Autodesk Inventor part; units mm, degrees
ref_plane "Work Plane1" through (0, 50.8, 0) normal (0, 1, 0) x (-1, 0, 0)
ref_plane "YZ Plane" through (0, 0, 0) normal (1, 0, 0) x (0, 1, 0)
ref_plane "XY Plane" through (0, 0, 0) normal (0, 0, 1) x (1, 0, 0)
sketch "Sketch1" plane through (0, 0, 0) normal (0, 0, 1) x (1, 0, 0)
  circle A0 centre (0, 0) radius 50.8
  circle A1 centre (0, 0) radius 47.625
  dimension "d0" = 101.6
  dimension "d1" = 95.25
extrude "Extrusion1" add sketch "Sketch1" along normal blind 711.2
ref_plane "Work Plane1" through (0, 50.8, 0) normal (0, 1, 0) x (-1, 0, 0)
sketch "Sketch3" plane through (0, 50.8, 0) normal (0, 1, 0) x (-1, 0, 0)
  line L0 (0, 0) -> (0, 111.76)
  line L1 (-4.7625, 111.76) -> (4.7625, 111.76)
  line L2 (4.7625, 111.76) -> (4.7625, 172.085)
  line L3 (4.7625, 172.085) -> (-4.7625, 172.085)
  line L4 (-4.7625, 172.085) -> (-4.7625, 111.76)
  dimension "d4" = 111.76
  dimension "d5" = 60.325
  dimension "d6" = 9.525
  dimension "d7" = 4.7625
extrude "Extrusion2" cut sketch "Sketch3" against normal blind 25.4
fillet "Fillet1" radius 4.7625 4 edges at (-4.7625, 48.9813, 111.76) (4.7625, 48.9813, 111.76) (4.7625, 48.9813, 172.085) (-4.7625, 48.9813, 172.085)
equation "\"d7\" = 0.5 * d6"
properties part number "PrimaryHullLexanTube_01" material "Polycarbonate, Clear"
Geometry check sheet. Reference: the model listing, model coordinates, mm. Give positions to 0.01 mm unless a question says otherwise; leave off trailing zeros. Loops run counter-clockwise (first coordinate to the right, second up) from the corner with the lowest first, then second, coordinate; pieces in that order, holes last. Notation, with made-up numbers: M 34.5,43.25 L 69.5,43.25 A22 cw 69.5,76.25 Z; hole C 27.25,3.5 d9. An arc over 180 degrees is marked long. Answer as a JSON object with one key per item and string values. Group by question number.
Item 1: Sectioned sample at C-C on z = 611.5. Record the boundary of the cut face in (x, y) (3 decimals).
Item 2: Mould release check, pull along X, two halves, no side actions. Record for faces 1 (the cylindrical face through (-37.794, 28.979, 350.622)), 2 (the flat face through (-15.3, 45.4, 0)), 3 (the cylindrical face through (-11.012, 49.592, 350.622)): pulls with the +X half, pulls with the -X half, needs draft (parallel to the pull), parting line crosses it, or undercut.
Item 3: Sectioned sample at B-B on x = 22. Record the boundary of the cut face in (y, z).
Item 4: Gauge pin test, flat ends, axial feed: pin 1 (8 mm diameter, centred on y = -8, z = 314, fed in from +X); pin 2 (1.5 mm diameter, centred on x = 9, z = 564, fed in from -Y); pin 3 (1 mm diameter, centred on x = -36.5, z = 463.5, fed in from -Y). Record the tip position at first contact, or that the pin passes through.
Item 5: Sectioned sample at A-A on y = 0. Record the boundary of the cut face in (x, z) (3 decimals).
Item 6: Material ranges on L1, parallel to X at y = 1, z = 293.5; L2, parallel to Y at x = 0, z = 398 (3 decimals); L3, parallel to Y at x = 0, z = 145.5 (3 decimals), recorded low to high.
Findings below:
{
 "1": {"outline": "C 0,0 d101.6; hole C 0,0 d95.25"},
 "2": {"face 1": "undercut", "face 2": "needs draft", "face 3": "parting line crosses it"},
 "3": {"outline": "M -45.79,0 L -42.24,0 L -42.24,711.2 L -45.79,711.2 Z; M 42.24,0 L 45.79,0 L 45.79,711.2 L 42.24,711.2 Z"},
 "4": {"pin 1": "x = 50.64", "pin 2": "y = -50.13", "pin 3": "y = -35.84"},
 "5": {"outline": "M -50.8,0 L -47.625,0 L -47.625,711.2 L -50.8,711.2 Z; M 47.625,0 L 50.8,0 L 50.8,711.2 L 47.625,711.2 Z"},
 "6": {"L1": "-50.79 to -47.61, 47.61 to 50.79", "L2": "-50.8 to -47.625, 47.625 to 50.8", "L3": "-50.8 to -47.625"}
}
